CAD build for the part. Positions are in the model's coordinates, mm. Face numbers are marked on the shaded views. A direction names the side the tool comes from. Round coordinates to 2 decimals unless told otherwise and drop trailing zeros. Order: outer loops, then holes, each group sorted by start corner. A loop starts at its lowest first (then second) coordinate and runs counter-clockwise, first axis right, second up. Notation, with made-up numbers: M 51,41 L 87,41 A16 ccw 87,69 Z; hole C -21,71.25 d11. An arc over 180 degrees is marked long. Answer as a JSON object with one key per item and string values.
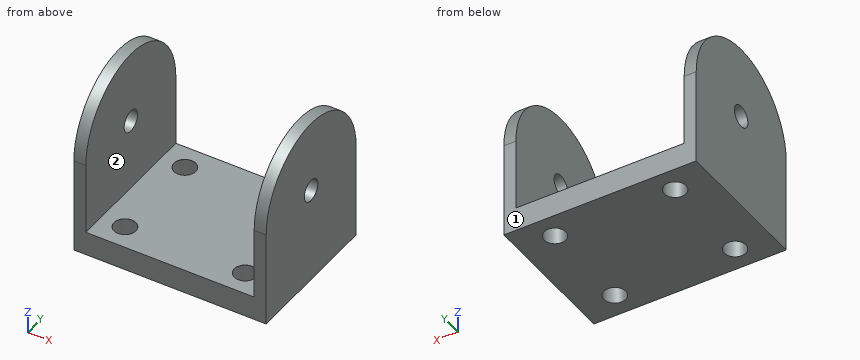
```python
from build123d import *

# Parameters (mm, degrees)
SKETCH1_W                      = 40
SKETCH1_H                      = 30
BOSS_EXTRUDE1_DEPTH            = 5
BOSS_EXTRUDE2_DEPTH            = 2.5
M4_CLEARANCE_HOLE2_D           = 4.5
M4_CLEARANCE_HOLE2_CSINK_D     = 4.55
M4_CLEARANCE_HOLE2_CSINK_ANGLE = 100


# Read off the part's stored shape, not the designer's step: M4 Clearance Hole1
with BuildPart() as part:
    # Sketch1 → Boss-Extrude1 (new body)
    with BuildSketch(Plane.XY):
        Rectangle(SKETCH1_W, SKETCH1_H)
    extrude(amount=BOSS_EXTRUDE1_DEPTH)

    # Sketch2 → Boss-Extrude2 (add)
    with BuildSketch(Plane(origin=(20, 0, 0), x_dir=(0, 0, -1), z_dir=(1, 0, 0))):
        with BuildLine():
            Line((-5, -15), (-5, 15))
            Line((-5, 15), (-20, 15))
            ThreePointArc((-20, 15), (-35, 0), (-20, -15))
            Line((-20, -15), (-5, -15))
        make_face()
    boss_extrude2 = extrude(amount=-BOSS_EXTRUDE2_DEPTH)

    # Mirror1: Boss-Extrude2 across plane
    add(boss_extrude2.mirror(Plane(origin=(0, 0, 0), x_dir=(0, 0, 1), z_dir=(1, 0, 0))))

    # M4 Clearance Hole1 outline → M4 Clearance Hole1 (revolve, cut)
    with BuildSketch(Plane(origin=(12.5, 10, 0), x_dir=(1, 0, 0), z_dir=(0, -1, 0))):
        Polygon((0, 0), (2.25, 0), (2.25, 4.979022509), (2.275, 5), (0, 5), align=None)
    revolve(axis=Axis((12.5, 10, 0), (0, 0, 1)), mode=Mode.SUBTRACT)

    # M4 Clearance Hole1 2 outline → M4 Clearance Hole1 2 (revolve, cut)
    with BuildSketch(Plane(origin=(-12.5, -10, 0), x_dir=(1, 0, 0), z_dir=(0, -1, 0))):
        Polygon((0, 0), (2.25, 0), (2.25, 4.979022509), (2.275, 5), (0, 5), align=None)
    revolve(axis=Axis((-12.5, -10, 0), (0, 0, 1)), mode=Mode.SUBTRACT)

    # M4 Clearance Hole1 3 outline → M4 Clearance Hole1 3 (revolve, cut)
    with BuildSketch(Plane(origin=(12.5, -10, 0), x_dir=(1, 0, 0), z_dir=(0, -1, 0))):
        Polygon((0, 0), (2.25, 0), (2.25, 4.979022509), (2.275, 5), (0, 5), align=None)
    revolve(axis=Axis((12.5, -10, 0), (0, 0, 1)), mode=Mode.SUBTRACT)

    # M4 Clearance Hole1 4 outline → M4 Clearance Hole1 4 (revolve, cut)
    with BuildSketch(Plane(origin=(-12.5, 10, 0), x_dir=(1, 0, 0), z_dir=(0, -1, 0))):
        Polygon((0, 0), (2.25, 0), (2.25, 4.979022509), (2.275, 5), (0, 5), align=None)
    revolve(axis=Axis((-12.5, 10, 0), (0, 0, 1)), mode=Mode.SUBTRACT)

    # M4 Clearance Hole2 (through all)
    with Locations(Plane(origin=(20, 0, 0), x_dir=(0, 0, -1), z_dir=(1, 0, 0))):
        with Locations((-20, 0)):
            CounterSinkHole(M4_CLEARANCE_HOLE2_D / 2, M4_CLEARANCE_HOLE2_CSINK_D / 2, counter_sink_angle=M4_CLEARANCE_HOLE2_CSINK_ANGLE)


solid = part.part
```
Item 1: 3-axis set-ups, long thin cutter, end or side, ignore diameter. For the marked faces 1 and 2: which of +Z, -Z, +X, -X, +Y, -Y reach the whole face in a straight line?
Worked answers:
{"face 1": "+Z, -Z, +X, -X, +Y", "face 2": "+Z, +Y, -Y"}
Item 2: Drop a flat-ended pin along its axis: pin 1 Ø7 at (x, y) = (-12.5, 10) entering from +Z. Give the stop position or say it passes through.
Worked answers:
{"pin 1": "stops at z = 5"}
Item 3: Saw through at C-C on z = 12. List the corners of the cut face in (x, y).
Worked answers:
{"outline": "M -20,-15 L -17.5,-15 L -17.5,15 L -20,15 Z; M 17.5,-15 L 20,-15 L 20,15 L 17.5,15 Z"}
Item 4: Saw through at B-B on x = 12.5. List the corners of the cut face in (y, z) (3 decimals).
Worked answers:
{"outline": "M -15,0 L -12.25,0 L -12.25,4.979 L -12.275,5 L -15,5 Z; M -7.75,0 L 7.75,0 L 7.75,4.979 L 7.725,5 L -7.725,5 L -7.75,4.979 Z; M 12.25,0 L 15,0 L 15,5 L 12.275,5 L 12.25,4.979 Z"}
Item 5: Saw through at A-A on y = 0. List the corners of the cut face in (x, z) (3 decimals), and give its area (4 significant figures).
Worked answers:
{"outline": "M -20,0 L 20,0 L 20,17.725 L 19.979,17.75 L 17.5,17.75 L 17.5,5 L -17.5,5 L -17.5,17.75 L -20,17.75 Z; M -20,22.25 L -17.5,22.25 L -17.5,35 L -20,35 Z; M 17.5,22.25 L 19.979,22.25 L 20,22.275 L 20,35 L 17.5,35 Z", "area": "327.5 mm2"}
Item 6: Saw through at D-D on y = -6.5. List the corners of the cut face in (x, z).
Worked answers:
{"outline": "M -20,0 L 20,0 L 20,33.52 L 17.5,33.52 L 17.5,5 L -17.5,5 L -17.5,33.52 L -20,33.52 Z"}
Item 7: Wall check: line 1 along Y through (x, z) = (12.5, 3.1); line 2 along X through (y, z) = (2, 22.5); line 3 along Z through (x, y) = (-2.5, -5.5). Give the ranges that are in metal, low to high. Write a range as [from, to].
Worked answers:
{"line 1": "y = [-15, -12.25], [-7.75, 7.75], [12.25, 15]", "line 2": "x = [-20, -17.5], [17.5, 20]", "line 3": "z = [0, 5]"}
